Input: part model. Units: mm. Frame: model coordinates. Round coordinates to 2 decimals unless told otherwise and drop trailing zeros. Order: outer loops, then holes, each group sorted by start corner. A loop starts at its lowest first (then second) coordinate and runs counter-clockwise, first axis right, second up.
Item 1: Cut plane D-D on x = -12. Output: boundary loops of the cut face in (y, z).
Item 2: First-contact query: pin 1 (0.6 mm diameter, centred on y = 12.5, z = 1, fed in from +X); pin 2 (1 mm diameter, centred on x = 1.5, z = 0, fed in from -Y). Flat tips, straight axial feed; report the tip coordinate or a pass-through.
Item 3: Line query: L1, parallel to Y at x = -24, z = 0.9; L2, parallel to Y at x = 23, z = 0.75; L3, parallel to Y at x = 11, z = 1.55. Output: solid intervals per line, ascending.
Item 4: Cut plane C-C on z = 0.45. Output: boundary loops of the cut face in (x, y), then the cut area to 3 significant figures.
Item 5: Cut plane A-A on x = -24. Output: boundary loops of the cut face in (y, z).
Item 6: Cut plane B-B on y = 39. Output: boundary loops of the cut face in (x, z).
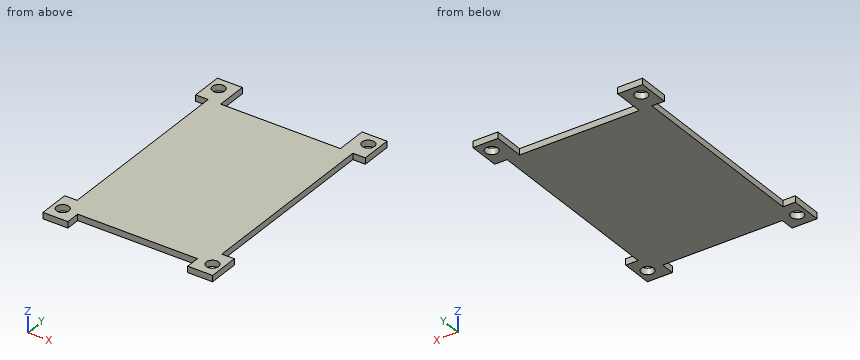
```python
from build123d import *

# Parameters (mm, degrees)
EXTRUSION1_DEPTH        = 2
ESQUISSE2_R             = 2
ENL_V_MAT_EXTRU_1_DEPTH = 3


with BuildPart() as part:
    # Esquisse1 → Extrusion1 (new body)
    with BuildSketch(Plane.XY):
        Polygon((-19.2, 33), (19.2, 33), (19.2, 43), (27.2, 43), (27.2, 33), (23.2, 33), (23.2, -27.5), (27.2, -27.5), (27.2, -37.5), (19.2, -37.5), (19.2, -33), (-19.2, -33), (-19.2, -37.5), (-27.2, -37.5), (-27.2, -27.5), (-23.2, -27.5), (-23.2, 33), (-27.2, 33), (-27.2, 43), (-19.2, 43), align=None)
    extrude(amount=EXTRUSION1_DEPTH)

    # Esquisse2 → Enlèv. mat.-Extru.1 (cut, through all)
    with BuildSketch(Plane.XY.offset(2)):
        with Locations((-24, 39)):
            Circle(ESQUISSE2_R)
        with Locations((24, 39)):
            Circle(ESQUISSE2_R)
        with Locations((-24, -33)):
            Circle(ESQUISSE2_R)
        with Locations((24, -33)):
            Circle(ESQUISSE2_R)
    extrude(amount=-ENL_V_MAT_EXTRU_1_DEPTH, mode=Mode.SUBTRACT)


solid = part.part
```
From the geometry:
1. outline: (-33, 0) - (33, 0) - (33, 2) - (-33, 2) - close
2. pin 1: stops at x = 23.2
2. pin 2: stops at y = -33
3. L1: y = -37.5 to -35, -31 to -27.5, 33 to 37, 41 to 43
3. L2: y = -37.5 to -34.73, -31.27 to 37.27, 40.73 to 43
3. L3: y = -33 to 33
4. outline: (-27.2, -37.5) - (-19.2, -37.5) - (-19.2, -33) - (19.2, -33) - (19.2, -37.5) - (27.2, -37.5) - (27.2, -27.5) - (23.2, -27.5) - (23.2, 33) - (27.2, 33) - (27.2, 43) - (19.2, 43) - (19.2, 33) - (-19.2, 33) - (-19.2, 43) - (-27.2, 43) - (-27.2, 33) - (-23.2, 33) - (-23.2, -27.5) - (-27.2, -27.5) - close; hole circle Ø4 at (-24, -33); hole circle Ø4 at (-24, 39); hole circle Ø4 at (24, -33); hole circle Ø4 at (24, 39)
4. area: 3,290 mm2
5. outline: (-37.5, 0) - (-35, 0) - (-35, 2) - (-37.5, 2) - close; (-31, 0) - (-27.5, 0) - (-27.5, 2) - (-31, 2) - close; (33, 0) - (37, 0) - (37, 2) - (33, 2) - close; (41, 0) - (43, 0) - (43, 2) - (41, 2) - close
6. outline: (-27.2, 0) - (-26, 0) - (-26, 2) - (-27.2, 2) - close; (-22, 0) - (-19.2, 0) - (-19.2, 2) - (-22, 2) - close; (19.2, 0) - (22, 0) - (22, 2) - (19.2, 2) - close; (26, 0) - (27.2, 0) - (27.2, 2) - (26, 2) - close
